Part print with two shaded views. Sizes in mm from the minimum x, y, z corner. A direction names the side the tool comes from. Round coordinates to 2 decimals unless told otherwise and drop trailing zeros. Write each loop counter-clockwise with the first axis right and the second up, starting at its lowest first coordinate (ties: lowest second). Pieces come first, ordered by that corner, then holes. Notation, with made-up numbers: (33.25, 18.25) -> (55.25, 18.25) arc R18 ccw to (55.25, 24.25) -> close; hole circle Ø6 at (73.5, 13). An arc over 180 degrees is marked (long way). Put each result on its own line as item: value. Start each with the question number.
1. Pull direction Y, two halves, no side cores. Call the marked faces 4, 5 and 6: pulls with the +Y half, pulls with the -Y half, needs draft (parallel to the pull), parting line crosses it, or undercut.
2. Saw through at A-A on x = 35. List the corners of the cut face in (y, z), and give its area (3 significant figures).
3. Saw through at D-D on x = 45. List the corners of the cut face in (y, z).
4. Flat gauge pins, fed straight in: P1, Ø4.5, axis at y = 25.5, z = 3.5, coming from the +X side; P2, Ø3, axis at x = 33.5, z = 28.5, coming from the +Y side; P3, Ø2.5, axis at y = 48.5, z = 63, coming from the -X side. Where does each tip first touch, or does it go through?
5. Drill centre lines: line 1 (Y direction, x = 35, z = 4); line 2 (Z direction, x = 15.5, y = 26); line 3 (X direction, y = 55, z = 60). Where is each one in solid material? Low to high. Write a range as from..to.
6. 3-axis set-ups, long thin cutter, end or side, ignore diameter. For the marked faces 1, 2 and 3: which of +Z, -Z, +X, -X, +Y, -Y reach the whole face in a straight line?
7. Saw through at B-B on y = 12. List the corners of the cut face in (x, z).
8. Saw through at C-C on y = 55. List the corners of the cut face in (x, z).
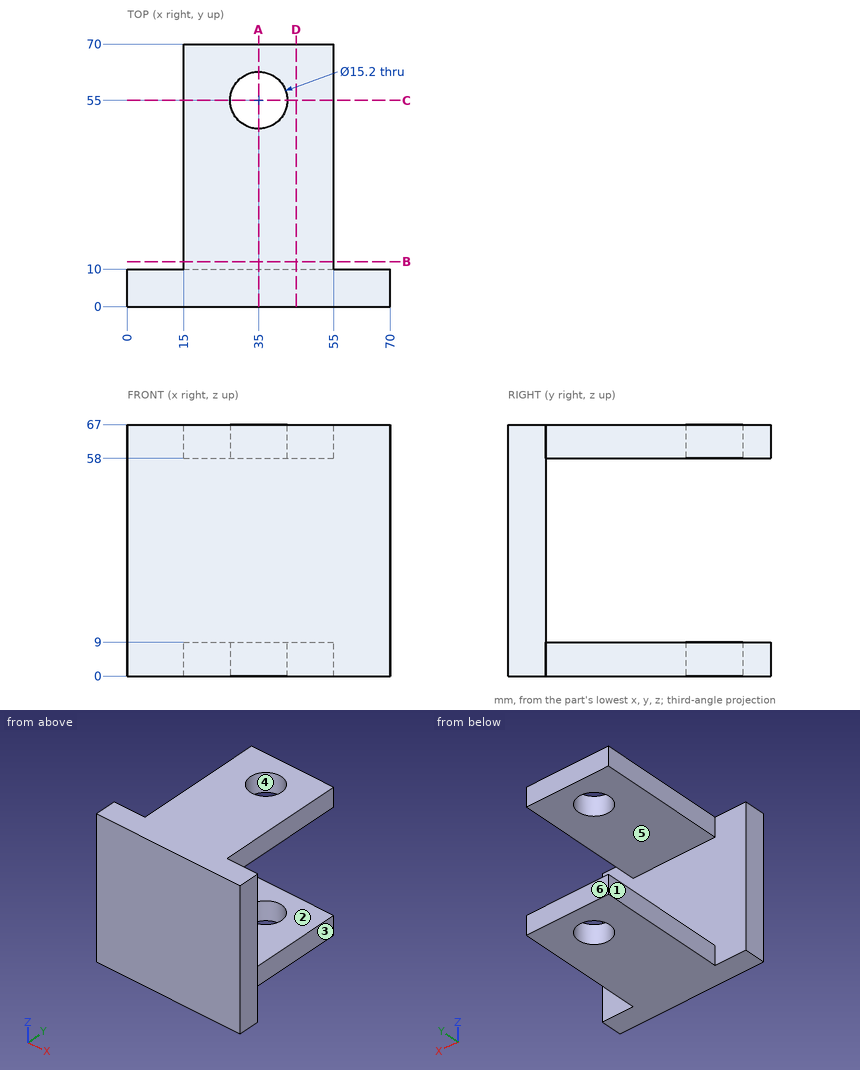
Return value:
1. face 4: undercut
1. face 5: needs draft
1. face 6: pulls with the +Y half
2. outline: (0, 0) -> (47.4, 0) -> (47.4, 9) -> (10, 9) -> (10, 58) -> (47.4, 58) -> (47.4, 67) -> (0, 67) -> close; (62.6, 0) -> (70, 0) -> (70, 9) -> (62.6, 9) -> close; (62.6, 58) -> (70, 58) -> (70, 67) -> (62.6, 67) -> close
2. area: 1,480 mm^2
3. outline: (0, 0) -> (70, 0) -> (70, 9) -> (10, 9) -> (10, 58) -> (70, 58) -> (70, 67) -> (0, 67) -> close
4. P1: stops at x = 55
4. P2: stops at y = 10
4. P3: stops at x = 15
5. line 1: y = 0..47.4, 62.6..70
5. line 2: z = 0..9, 58..67
5. line 3: x = 15..27.4, 42.6..55
6. face 1: +Z, -Z, -X, +Y
6. face 2: +X, -X, +Y
6. face 3: +Z, -Z, +X, +Y
7. outline: (15, 0) -> (55, 0) -> (55, 9) -> (15, 9) -> close; (15, 58) -> (55, 58) -> (55, 67) -> (15, 67) -> close
8. outline: (15, 0) -> (27.4, 0) -> (27.4, 9) -> (15, 9) -> close; (15, 58) -> (27.4, 58) -> (27.4, 67) -> (15, 67) -> close; (42.6, 0) -> (55, 0) -> (55, 9) -> (42.6, 9) -> close; (42.6, 58) -> (55, 58) -> (55, 67) -> (42.6, 67) -> close
